```python
from build123d import *

# Parameters (mm, degrees)
F1_DEPTH = 101.6
F2_W     = 1257.021352
F2_H     = 189.658009
F3_DEPTH = 304.801
F4_DEPTH = 152.401


with BuildPart() as f1:
    # F0 (on Top) → F1 (new body)
    with BuildSketch(Plane.XY):
        with BuildLine():
            ThreePointArc((-81.28, 251.036195), (-50.828259, 188.00114), (-84.666667, 126.717463))
            ThreePointArc((-84.666667, 126.717463), (-145.838098, -44.238098), (0, -152.4))
            Line((0, -152.4), (152.4, -152.4))
            ThreePointArc((152.4, -152.4), (298.238098, -44.238098), (237.066667, 126.717463))
            ThreePointArc((237.066667, 126.717463), (203.838207, 180.234678), (222.25, 240.477758))
            ThreePointArc((222.25, 240.477758), (226.166681, 268.126854), (202.32325, 282.663142))
            ThreePointArc((202.32325, 282.663142), (131.315454, 309.943826), (101.6, 379.96764))
            Line((101.6, 379.96764), (101.6, 850.476195))
            Line((101.6, 850.476195), (140.308257, 883.505244))
            ThreePointArc((140.308257, 883.505244), (148.047216, 895.194332), (148.406537, 909.208509))
            Line((148.406537, 909.208509), (109.953977, 1056.373323))
            ThreePointArc((109.953977, 1056.373323), (90.045146, 1074.919879), (64.781823, 1064.815382))
            Line((64.781823, 1064.815382), (42.783839, 1034.330968))
            Line((42.783839, 1034.330968), (34.39404, 1021.281634))
            ThreePointArc((34.39404, 1021.281634), (32.491534, 1017.732173), (31.173938, 1013.926632))
            Line((31.173938, 1013.926632), (3.993463, 909.208509))
            ThreePointArc((3.993463, 909.208509), (4.352784, 895.194332), (12.091743, 883.505244))
            Line((12.091743, 883.505244), (50.8, 850.476195))
            Line((50.8, 850.476195), (50.8, 393.276195))
            ThreePointArc((50.8, 393.276195), (35.921024, 357.355171), (0, 342.476195))
            Line((0, 342.476195), (-50.8, 342.476195))
            ThreePointArc((-50.8, 342.476195), (-98.993112, 307.740566), (-81.28, 251.036195))
        make_face()
    extrude(amount=F1_DEPTH)

    # F2 (on Right) → F3 (cut, through all)
    with BuildSketch(Plane.YZ):
        with Locations((456.159748, 22.18328)):
            Rectangle(F2_W, F2_H)
        with BuildLine():
            ThreePointArc((1056.942703, 89.788765), (1049.503216, 71.828253), (1031.542703, 64.388765))
            Line((1031.542703, 64.388765), (422.418403, 64.388765))
            ThreePointArc((422.418403, 64.388765), (407.414851, 59.48397), (398.205736, 46.663839))
            ThreePointArc((398.205736, 46.663839), (394.189746, 38.935854), (387.799281, 33.01877))
            Line((387.799281, 33.01877), (369.241137, 21.001137))
            ThreePointArc((369.241137, 21.001137), (362.633132, 17.962589), (355.434925, 16.92128))
            Line((355.434925, 16.92128), (-86.235178, 16.92128))
            ThreePointArc((-86.235178, 16.92128), (-103.426242, 19.918484), (-118.588758, 28.556425))
            Line((-118.588758, 28.556425), (-144.24981, 49.754688))
            ThreePointArc((-144.24981, 49.754688), (-151.051819, 58.514234), (-153.47302, 69.337115))
            Line((-153.47302, 69.337115), (-153.47302, 76.600858))
            ThreePointArc((-153.47302, 76.600858), (-151.357661, 86.749034), (-145.363926, 95.206893))
            ThreePointArc((-145.363926, 95.206893), (-137.361903, 100.24143), (-128.07302, 102.000858))
            Line((-128.07302, 102.000858), (1050.592703, 102.000858))
            ThreePointArc((1050.592703, 102.000858), (1055.082831, 100.140986), (1056.942703, 95.650858))
            Line((1056.942703, 95.650858), (1056.942703, 89.788765))
        make_face(mode=Mode.SUBTRACT)
    extrude(amount=F3_DEPTH, mode=Mode.SUBTRACT)

    # F2 (on Right) → F4 (cut, through all)
    with BuildSketch(Plane.YZ):
        with Locations((456.159748, 22.18328)):
            Rectangle(F2_W, F2_H)
        with BuildLine():
            ThreePointArc((1056.942703, 89.788765), (1049.503216, 71.828253), (1031.542703, 64.388765))
            Line((1031.542703, 64.388765), (422.418403, 64.388765))
            ThreePointArc((422.418403, 64.388765), (407.414851, 59.48397), (398.205736, 46.663839))
            ThreePointArc((398.205736, 46.663839), (394.189746, 38.935854), (387.799281, 33.01877))
            Line((387.799281, 33.01877), (369.241137, 21.001137))
            ThreePointArc((369.241137, 21.001137), (362.633132, 17.962589), (355.434925, 16.92128))
            Line((355.434925, 16.92128), (-86.235178, 16.92128))
            ThreePointArc((-86.235178, 16.92128), (-103.426242, 19.918484), (-118.588758, 28.556425))
            Line((-118.588758, 28.556425), (-144.24981, 49.754688))
            ThreePointArc((-144.24981, 49.754688), (-151.051819, 58.514234), (-153.47302, 69.337115))
            Line((-153.47302, 69.337115), (-153.47302, 76.600858))
            ThreePointArc((-153.47302, 76.600858), (-151.357661, 86.749034), (-145.363926, 95.206893))
            ThreePointArc((-145.363926, 95.206893), (-137.361903, 100.24143), (-128.07302, 102.000858))
            Line((-128.07302, 102.000858), (1050.592703, 102.000858))
            ThreePointArc((1050.592703, 102.000858), (1055.082831, 100.140986), (1056.942703, 95.650858))
            Line((1056.942703, 95.650858), (1056.942703, 89.788765))
        make_face(mode=Mode.SUBTRACT)
    extrude(amount=-F4_DEPTH, mode=Mode.SUBTRACT)


solid = f1.part
```
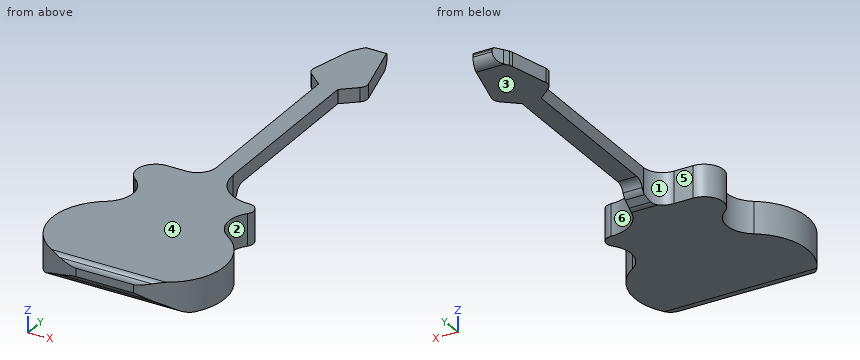
For this review, take the finished solid that the model builds, in its own axes (mm). Face numbers are marked on the shaded views. A direction names the side the tool comes from. Round coordinates to 2 decimals unless told otherwise and drop trailing zeros. Order: outer loops, then holes, each group sorted by start corner. A loop starts at its lowest first (then second) coordinate and runs counter-clockwise, first axis right, second up. Notation, with made-up numbers: (70.5, -12.75) -> (104.5, -12.75) arc R10 cw to (104.5, -7.75) -> close; hole circle Ø8 at (25.25, -26). An arc over 180 degrees is marked (long way). Use a Markdown table: item, result.
Item 1: Draft analysis for pull direction Y (two halves, no side actions). For the marked faces 4, 5 and 6, state which applies: +Y half, -Y half, draft (parallel to the pull), parting line (faces both ways), or undercut.
Resolved:
| item | result |
|---|---|
| face 4 | draft |
| face 5 | +Y half |
| face 6 | undercut |
Item 2: Take a section at A-A (x = 80.5). State the section outline as (y, z) points.
Resolved:
| item | result |
|---|---|
| outline | (-152.4, 62.03) arc R25.4 ccw to (-144.25, 49.75) -> (-118.59, 28.56) arc R50.8 ccw to (-86.24, 16.92) -> (355.43, 16.92) arc R25.4 ccw to (369.24, 21) -> (387.8, 33.02) arc R25.4 ccw to (398.21, 46.66) arc R25.4 cw to (422.42, 64.39) -> (1031.54, 64.39) arc R25.4 ccw to (1056.94, 89.79) -> (1056.94, 95.65) arc R6.35 ccw to (1052.81, 101.6) -> (-132.57, 101.6) arc R25.4 ccw to (-145.36, 95.21) arc R25.4 ccw to (-152.4, 83.91) -> close |
Item 3: Take a section at C-C (x = 183.5). State the section outline as (y, z) points, plus the area to 3 significant figures.
Resolved:
| item | result |
|---|---|
| outline | (-149.19, 55.23) arc R25.4 ccw to (-144.25, 49.75) -> (-118.59, 28.56) arc R50.8 ccw to (-86.24, 16.92) -> (283.84, 16.92) -> (283.84, 101.6) -> (-132.57, 101.6) arc R25.4 ccw to (-145.36, 95.21) arc R25.4 ccw to (-149.19, 90.71) -> close |
| area | 35,700 mm² |
Item 4: For line 1 along X through (y, z) = (729, 74); line 2 along Y through (x, z) = (-36, 95); line 3 along Z through (x, y) = (87, 916.5), list the stretches that pass through material, from the lowest coordinate up. Write a range as [from, to].
Resolved:
| item | result |
|---|---|
| line 1 | x = [50.8, 101.6] |
| line 2 | y = [-145.58, 342.48] |
| line 3 | z = [64.39, 101.6] |
Item 5: Take a section at B-B (y = 739). State the section outline as (x, z) points.
Resolved:
| item | result |
|---|---|
| outline | (50.8, 64.39) -> (101.6, 64.39) -> (101.6, 101.6) -> (50.8, 101.6) -> close |
Item 6: Machinability: for the marked faces 1, 2 and 3, which of the approach directions +Z, -Z, +X, -X, +Y, -Y give a long, thin tool a straight path to every point of the face, cutting with its end or side? Answer none if there is none.
Resolved:
| item | result |
|---|---|
| face 1 | +Z, -Z, -X |
| face 2 | +Z, -Z, +X |
| face 3 | -Z, +X, -X, +Y |
Item 7: Take a section at D-D (y = 148). State the section outline as (x, z) points.
Resolved:
| item | result |
|---|---|
| outline | (-63.47, 16.92) -> (215.87, 16.92) -> (215.87, 101.6) -> (-63.47, 101.6) -> close |
Item 8: For pin 1 (1.5 mm diameter, centred on y = 477, z = 68.5, fed in from +X); pin 2 (4 mm diameter, centred on x = -43.5, z = 69, fed in from -Y); pin 3 (5 mm diameter, centred on y = 106, z = 55.5, fed in from -X), all flat-tipped, find the tip position at first contact; note any pin that passes through.
Resolved:
| item | result |
|---|---|
| pin 1 | stops at x = 101.6 |
| pin 2 | stops at y = -146.64 |
| pin 3 | stops at x = -111.86 |
